Here's the drawing with two shaded views (mm, measured from the low corner). I have some questions. A direction names the side the tool comes from. Round coordinates to 2 decimals unless told otherwise and drop trailing zeros. Loops run counter-clockwise (first coordinate to the right, second up) from the corner with the lowest first, then second, coordinate; pieces in that order, holes last. Notation, with made-up numbers: (-5.5, 68) -> (50.5, 68) arc R15 ccw to (50.5, 88) -> close; hole circle Ø5 at (-4.75, 13). An arc over 180 degrees is marked (long way). Write each question's results on one line, items separated by ' | '. Start each with the question number.
1) Which directions (+Z, -Z, +X, -X, +Y, -Y) give clear straight access to the entire face, cutting with the end or side of a thin tool? Please do the marked faces 1, 2 and 3.
2) If I drill on probe 1 along Y at (x, z) = (3, 20.75) (1 decimal); probe 2 along Y at (x, z) = (17.5, 16.25); probe 3 along X at (y, z) = (17, 18.25), over which ranges is the centre line in solid material (lowest first)?
3) Imagine slicing it at C-C, the plane z = 10. List the corners of the cut face in (x, y) for me.
4) For P1, Ø6, axis at x = 14, z = 10, coming from the +Y side; P2, Ø10.5, axis at x = 21, y = 13.5, coming from the -Z side; P3, Ø3, axis at x = 5.5, y = 30.5, coming from the +Z side; P4, Ø6, axis at x = 25.5, z = 7.5, coming from the +Y side, each with a flat end and sliding along its axis, tell me the tip position at first contact or that it passes through.
5) Imagine slicing it at A-A, the plane y = 17.5. List the corners of the cut face in (x, z) for me.
6) We'd pull the mould along Y, two halves only. Please class the marked faces 4, 5 and 6: pulls with the +Y half, pulls with the -Y half, needs draft (parallel to the pull), parting line crosses it, or undercut.
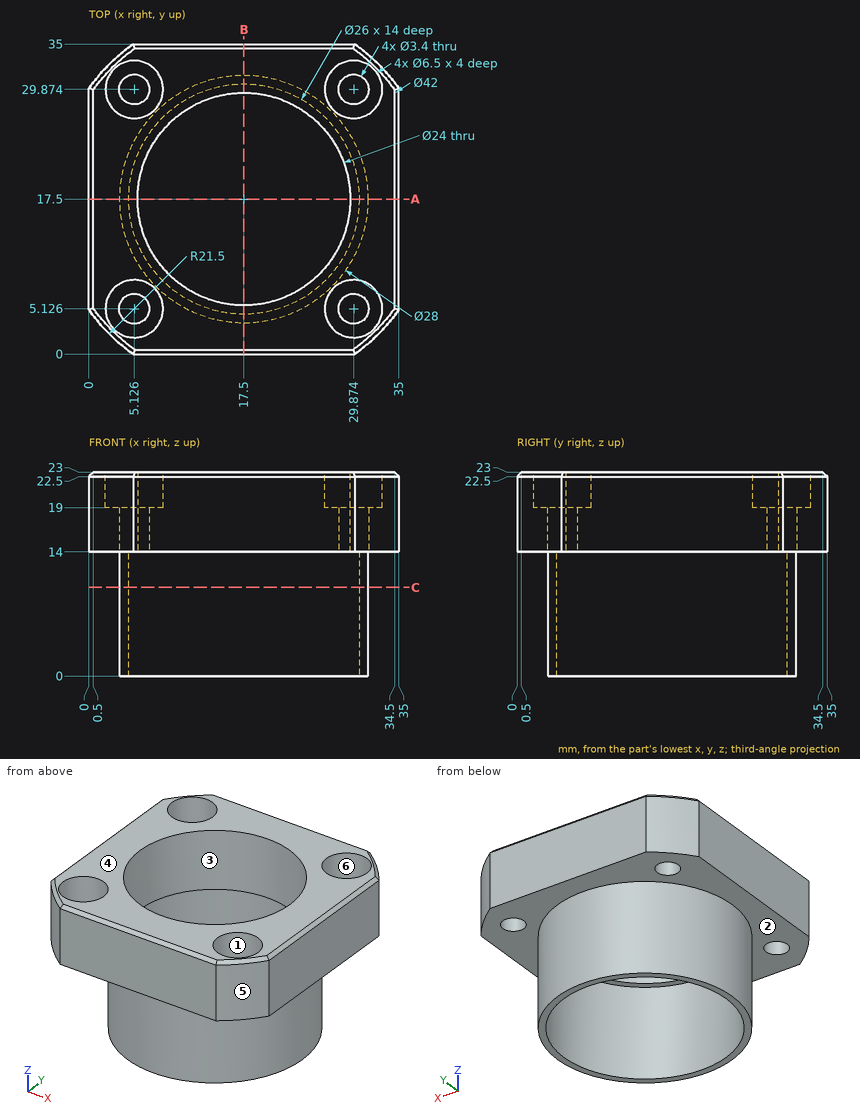
Checked values:
1) face 1: +Z | face 2: -Z | face 3: +Z, -Z
2) probe 1: 1.6 to 2.7, 7.6 to 27.4, 32.3 to 33.4 | probe 2: 0 to 5.5, 29.5 to 35 | probe 3: 0 to 5.51, 29.49 to 35
3) outline: circle Ø28 at (17.5, 17.5); hole circle Ø26 at (17.5, 17.5)
4) P1: y = 31.49 | P2: through | P3: z = 19 | P4: y = 30.58
5) outline: (0, 14) -> (3.5, 14) -> (3.5, 0) -> (4.5, 0) -> (4.5, 14) -> (5.5, 14) -> (5.5, 23) -> (0.5, 23) -> (0, 22.5) -> close; (29.5, 14) -> (30.5, 14) -> (30.5, 0) -> (31.5, 0) -> (31.5, 14) -> (35, 14) -> (35, 22.5) -> (34.5, 23) -> (29.5, 23) -> close
6) face 4: needs draft | face 5: pulls with the -Y half | face 6: undercut
